Input: dimensioned drawing with shaded views. Units: mm. Origin: part minimum x, y, z. Give positions to 0.01 mm unless a question says otherwise; leave off trailing zeros. Loops run counter-clockwise (first coordinate to the right, second up) from the corner with the lowest first, then second, coordinate; pieces in that order, holes last. Notation, with made-up numbers: (41.25, 56.25) -> (61.25, 56.25) arc R14 cw to (61.25, 83.25) -> close; hole circle Ø10 at (50, 36.25). An arc over 180 degrees is marked (long way). Answer as a JSON object with one key per item and string values.
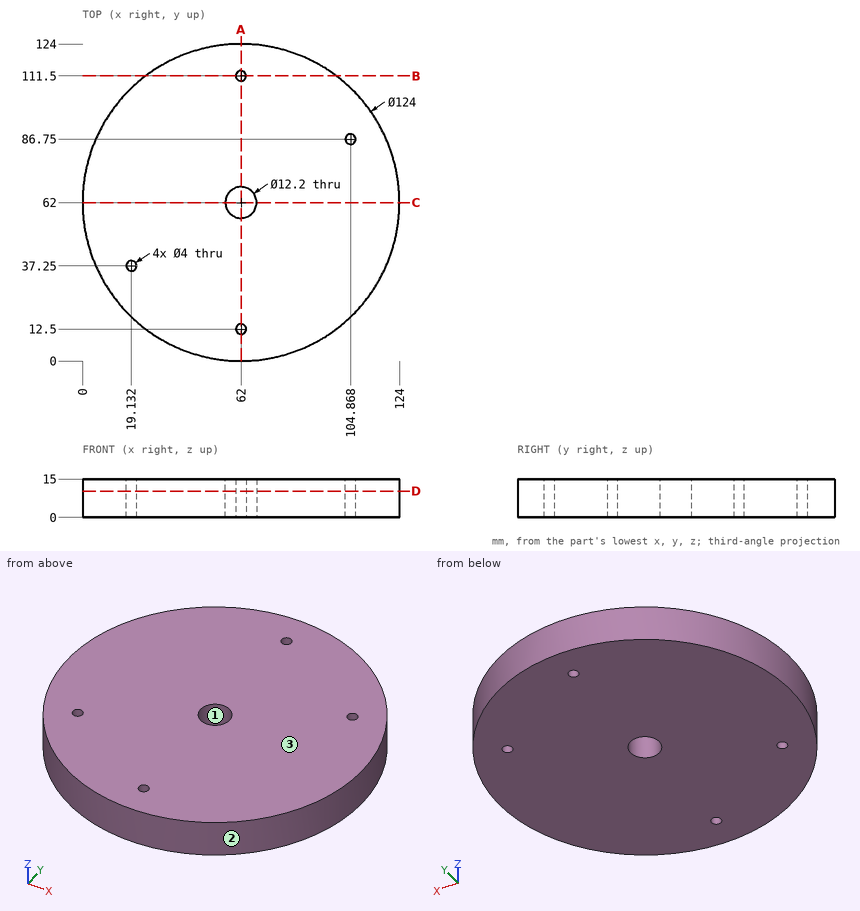
Q1. Section B-B, the plane y = 111.5. Return the cut outline in (x, z).
Evaluation:
{"outline": "(24.67, 0) -> (60, 0) -> (60, 15) -> (24.67, 15) -> close; (64, 0) -> (99.33, 0) -> (99.33, 15) -> (64, 15) -> close"}
Q2. Section D-D, the plane z = 10.25. Return the cut outline in (x, y).
Evaluation:
{"outline": "circle Ø124 at (62, 62); hole circle Ø4 at (19.13, 37.25); hole circle Ø12.2 at (62, 62); hole circle Ø4 at (62, 12.5); hole circle Ø4 at (62, 111.5); hole circle Ø4 at (104.87, 86.75)"}
Q3. Pin query (flat end, axial travel): pin 1 (2 mm diameter, centred on y = 104, z = 9.5, fed in from -X); pin 2 (11 mm diameter, centred on x = 62, y = 62, fed in from -Z); pin 3 (5 mm diameter, centred on y = 87.5, z = 5, fed in from -X). Return the tip coordinate at first contact, or that it passes through.
Evaluation:
{"pin 1": "stops at x = 15.49", "pin 2": "passes through", "pin 3": "stops at x = 4.42"}
Q4. Ray query, line 1 along Y through (x, z) = (62, 3.25); line 2 along X through (y, z) = (110, 4); line 3 along X through (y, z) = (111.5, 3.75). Return the intervals inside material, ascending.
Evaluation:
{"line 1": "y = 0 to 10.5, 14.5 to 55.9, 68.1 to 109.5, 113.5 to 124", "line 2": "x = 22.76 to 60.68, 63.32 to 101.24", "line 3": "x = 24.67 to 60, 64 to 99.33"}
Q5. Section A-A, the plane x = 62. Return the cut outline in (y, z), then the cut area to 3 significant figures.
Evaluation:
{"outline": "(0, 0) -> (10.5, 0) -> (10.5, 15) -> (0, 15) -> close; (14.5, 0) -> (55.9, 0) -> (55.9, 15) -> (14.5, 15) -> close; (68.1, 0) -> (109.5, 0) -> (109.5, 15) -> (68.1, 15) -> close; (113.5, 0) -> (124, 0) -> (124, 15) -> (113.5, 15) -> close", "area": "1,560 mm2"}
Q6. Section C-C, the plane y = 62. Return the cut outline in (x, z), then the cut area to 3 significant figures.
Evaluation:
{"outline": "(0, 0) -> (55.9, 0) -> (55.9, 15) -> (0, 15) -> close; (68.1, 0) -> (124, 0) -> (124, 15) -> (68.1, 15) -> close", "area": "1,680 mm2"}
Q7. Draft query along Y for the marked faces 1, 2 and 3. Return one class per face: +Y half, -Y half, draft (parallel to the pull), parting line (faces both ways), or undercut.
Evaluation:
{"face 1": "undercut", "face 2": "parting line", "face 3": "draft"}
